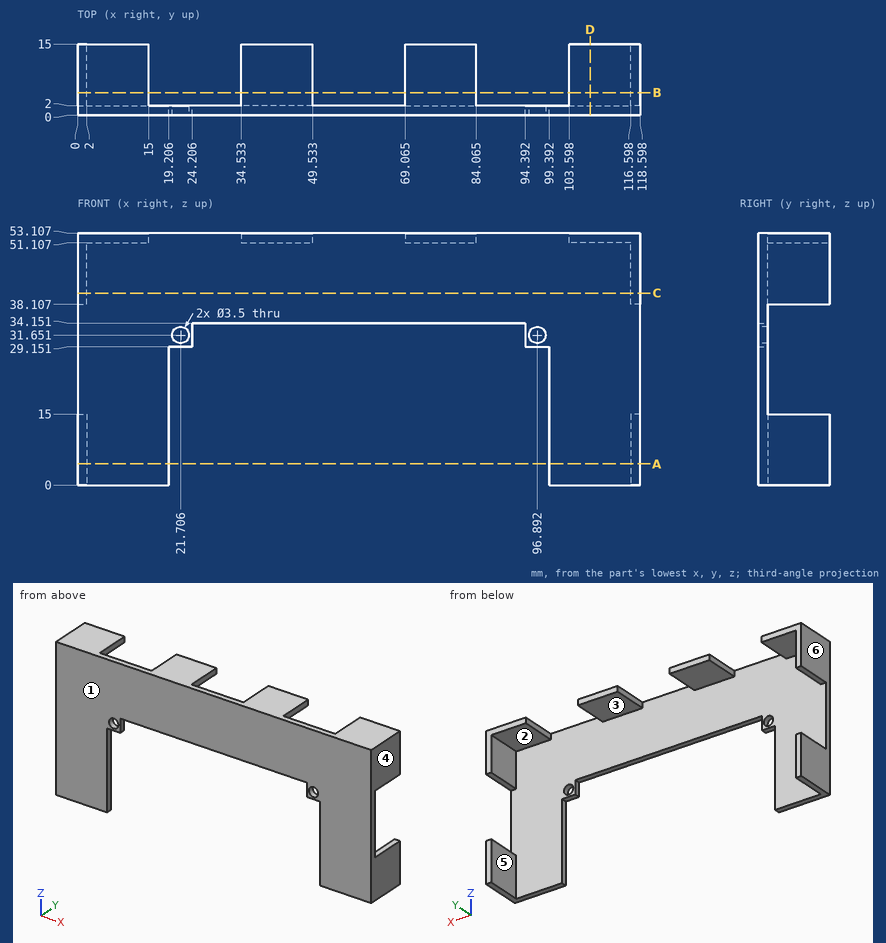
Geometry check sheet. Reference: drawing and pictorial views, mm from the part's lowest x, y, z. A direction names the side the tool comes from. Coordinates: 2 decimals unless noted, no trailing zeros. Write each loop counter-clockwise with the first axis right and the second up, starting at its lowest first coordinate (ties: lowest second). Pieces come first, ordered by that corner, then holes. Notation, with made-up numbers: M -8,-7 L 26,-7 A14 ccw 26,18 Z; hole C 65,32 d11. An arc over 180 degrees is marked long. One line per question, with ' | ' between items.
1) Sectioned sample at D-D on x = 108. Record the cut outline in (y, z), then the cut area to 3 significant figures.
Solutions:
outline: M 0,0 L 2,0 L 2,51.11 L 15,51.11 L 15,53.11 L 0,53.11 Z | area: 132 mm^2
2) Access from +Z, -Z, +X, -X, +Y, -Y to the whole of each face (thin tool, end or side, straight path). Record for the marked faces 1 and 2.
Solutions:
face 1: +Z, -Z, +X, -X, -Y | face 2: -Z, +Y
3) Sectioned sample at B-B on y = 4.75. Record the cut outline in (x, z) (1 decimal), then the cut area to 3 significant figures.
Solutions:
outline: M 0,0 L 2,0 L 2,15 L 0,15 Z; M 0,38.1 L 2,38.1 L 2,51.1 L 15,51.1 L 15,53.1 L 0,53.1 Z; M 34.5,51.1 L 49.5,51.1 L 49.5,53.1 L 34.5,53.1 Z; M 69.1,51.1 L 84.1,51.1 L 84.1,53.1 L 69.1,53.1 Z; M 103.6,51.1 L 116.6,51.1 L 116.6,38.1 L 118.6,38.1 L 118.6,53.1 L 103.6,53.1 Z; M 116.6,0 L 118.6,0 L 118.6,15 L 116.6,15 Z | area: 232 mm^2
4) Material ranges on L1, parallel to X at y = 3.5, z = 3.5; L2, parallel to Y at x = 87, z = 46; L3, parallel to X at y = 1, z = 24.5, recorded low to high.
Solutions:
L1: 0 to 2, 116.6 to 118.6 | L2: 0 to 2 | L3: 0 to 19.21, 99.39 to 118.6
5) Depth check by flat-ended pin: pin 1 Ø0.6 at (x, y) = (21.5, 0.5) entering from -Z; pin 2 Ø1.6 at (y, z) = (9, 52) entering from -X; pin 3 Ø4 at (x, y) = (43.5, 7) entering from -Z; pin 4 Ø3 at (x, z) = (21.71, 31.65) entering from +Y. Enter the tip coordinate at first touch or a pass-through.
Solutions:
pin 1: z = 29.15 | pin 2: x = 0 | pin 3: z = 51.11 | pin 4: through
6) Sectioned sample at C-C on z = 40.5. Record the cut outline in (x, y).
Solutions:
outline: M 0,0 L 118.6,0 L 118.6,15 L 116.6,15 L 116.6,2 L 2,2 L 2,15 L 0,15 Z
7) Sectioned sample at A-A on z = 4.5. Record the cut outline in (x, y), then the cut area to 3 significant figures.
Solutions:
outline: M 0,0 L 19.21,0 L 19.21,2 L 2,2 L 2,15 L 0,15 Z; M 99.39,0 L 118.6,0 L 118.6,15 L 116.6,15 L 116.6,2 L 99.39,2 Z | area: 129 mm^2
8) Release check for a two-part mould opening along X. For the marked faces 3, 4, 5 and 6 record: +X half, -X half, draft (parallel to the pull), parting line (faces both ways), or undercut.
Solutions:
face 3: undercut | face 4: +X half | face 5: undercut | face 6: -X half
